Geometry check sheet. Reference: the model listing, model coordinates, mm. A direction names the side the tool comes from. Round coordinates to 2 decimals unless told otherwise and drop trailing zeros. Loops run counter-clockwise (first coordinate to the right, second up) from the corner with the lowest first, then second, coordinate; pieces in that order, holes last. Notation, with made-up numbers: M -21,8.5 L 30,8.5 A26 cw 30,31.5 Z; hole C 42,21.25 d10. An arc over 180 degrees is marked long. Write item = value, one per line.
from build123d import *

# Parameters (mm, degrees)
F0_W     = 25.4
F0_H     = 6.35
F1_DEPTH = 38.1
F2_W     = 12.7
F2_H     = 19.05
F3_DEPTH = 25.4
F5_DEPTH = 12.7


with BuildPart() as f1:
    # F0 (on Front) → F1 (new body)
    with BuildSketch(Plane.XZ):
        with Locations((12.7, 3.175)):
            Rectangle(F0_W, F0_H)
        Polygon((0, 25.4), (0, 6.35), (25.4, 6.35), align=None)
    extrude(amount=-F1_DEPTH)

    # F2 (on face) → F3 (cut)
    with BuildSketch(Plane(origin=(0, 0, 0), x_dir=(0, -1, 0), z_dir=(-1, 0, 0))):
        with Locations((-6.35, 15.875)):
            Rectangle(F2_W, F2_H)
    extrude(amount=-F3_DEPTH, mode=Mode.SUBTRACT)

    # F4 (on face) → F5 (cut)
    with BuildSketch(Plane.XZ.offset(-12.7)):
        Polygon((0, 25.4), (0, 19.05), (8.466667, 19.05), align=None)
    extrude(amount=-F5_DEPTH, mode=Mode.SUBTRACT)


solid = f1.part
(1) Sectioned sample at A-A on x = 8. Record the cut outline in (y, z), then the cut area to 3 significant figures.
Result set:
outline = M 0,0 L 38.1,0 L 38.1,19.4 L 25.4,19.4 L 25.4,19.05 L 12.7,19.05 L 12.7,6.35 L 0,6.35 Z
area = 569 mm2
(2) Tool access check on faces 1 (the flat face through (0, 23, 10)), 2 (the flat face through (13, 6, 6.35)). Record the directions out of +Z, -Z, +X, -X, +Y, -Y that give a thin tool (end or side, any length) a straight path to the whole face; none if there is none.
Result set:
face_1 = +Z, -Z, -X, +Y, -Y
face_2 = +Z, +X, -X, -Y
(3) Sectioned sample at D-D on x = 12. Record the cut outline in (y, z), then the cut area to 3 significant figures.
Result set:
outline = M 0,0 L 38.1,0 L 38.1,16.4 L 12.7,16.4 L 12.7,6.35 L 0,6.35 Z
area = 497 mm2
(4) Material ranges on line 1 along Z through (x, y) = (5.5, 8); line 2 along Y through (x, z) = (1.5, 16.5), recorded low to high. Write a range as from..to.
Result set:
line_1 = 0..6.35
line_2 = 12.7..38.1
(5) Sectioned sample at B-B on y = 28. Record the cut outline in (x, z), then the cut area to 3 significant figures.
Result set:
outline = M 0,0 L 25.4,0 L 25.4,6.35 L 0,25.4 Z
area = 403 mm2
(6) Sectioned sample at C-C on z = 13.25. Record the cut outline in (x, y).
Result set:
outline = M 0,12.7 L 16.2,12.7 L 16.2,38.1 L 0,38.1 Z
(7) Depth check by flat-ended pin: pin 1 Ø12 at (x, y) = (8.5, 32) entering from +Z (3 decimals); pin 2 Ø10 at (x, z) = (17, 12.5) entering from -Y; pin 3 Ø3 at (x, y) = (5.5, 20.5) entering from +Z. Enter the tip coordinate at first touch or a pass-through.
Result set:
pin_1 = 23.525
pin_2 = 12.7
pin_3 = 19.05
